The drawing under review shows one solid part. Ordinate dimensions are in mm from its lowest x, y, z. A direction names the side the tool comes from. Round coordinates to 2 decimals unless told otherwise and drop trailing zeros. Loops run counter-clockwise (first coordinate to the right, second up) from the corner with the lowest first, then second, coordinate; pieces in that order, holes last. Notation, with made-up numbers: (69.5, 52.5) -> (98.5, 52.5) arc R24 cw to (98.5, 85.5) -> close; hole circle Ø8 at (0.25, 60.5). An arc over 180 degrees is marked (long way). Use a Markdown table: item, result. Add a question column.
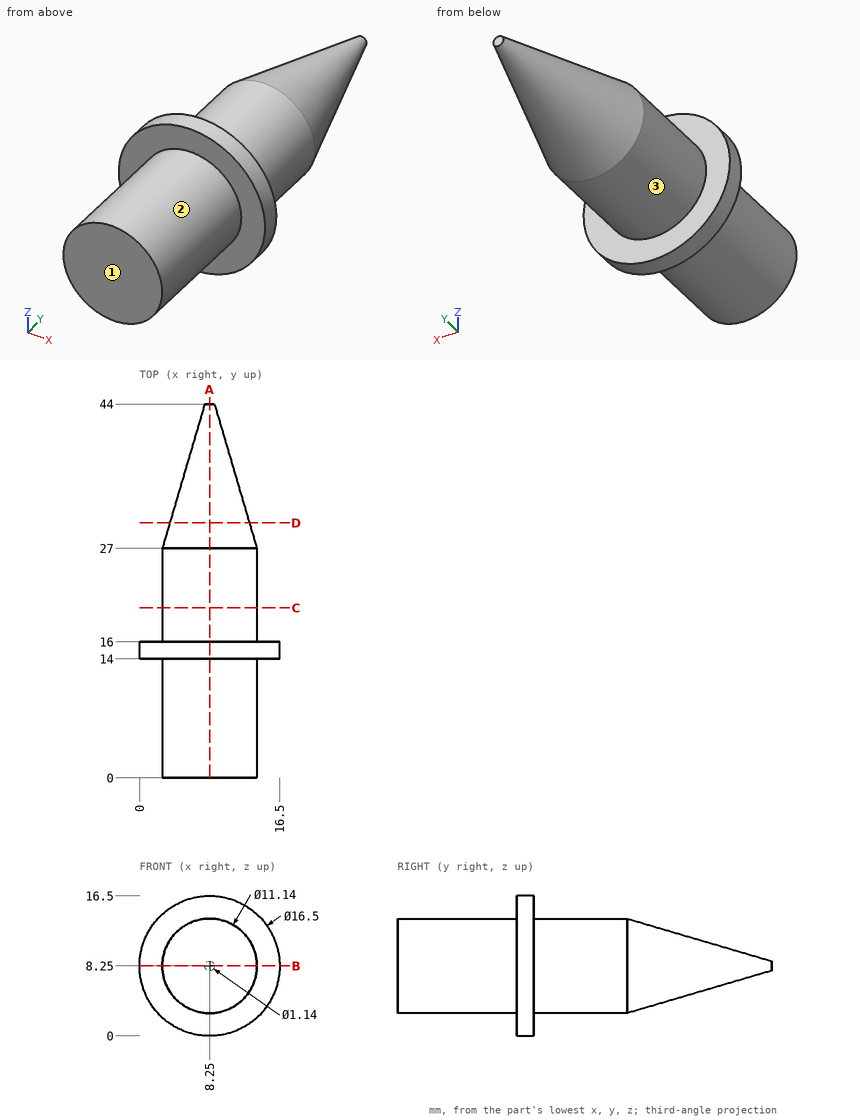
1. Insertion check: P1, Ø2, axis at x = 11, z = 2, coming from the -Y side; P2, Ø6, axis at y = 31.5, z = 2.5, coming from the -X side. Each pin has a flat end and moves straight along its axis. Give the tip position at first contact, or say it passes through.
2. For the marked faces 1, 2 and 3, list the 3-axis set-ups (+Z, -Z, +X, -X, +Y, -Y) from which the entire face can be reached by the end or side of a thin tool; tool diameter is ignored.
3. To check wall thickness, follow probe 1 along Y at (x, z) = (5, 15.25); probe 2 along X at (y, z) = (33, 9.5); probe 3 along X at (y, z) = (12, 5.75). State the ranges of each line that lie inside material, in increasing order. Write a range as from..to.
4. Consider section C-C on y = 20. State the section outline as (x, z) points.
5. Consider section A-A on x = 8.25. State the section outline as (y, z) points.
6. Consider section B-B on z = 8.25. State the section outline as (x, y) points, plus the area to 3 significant figures.
7. Consider section D-D on y = 30. State the section outline as (x, z) points.
Verdict:
| question | item | result |
|---|---|---|
| 1 | P1 | stops at y = 14 |
| 1 | P2 | stops at x = 4.76 |
| 2 | face 1 | +Z, -Z, +X, -X, -Y |
| 2 | face 2 | -Y |
| 2 | face 3 | +Y |
| 3 | probe 1 | y = 14..16 |
| 3 | probe 2 | x = 4.66..11.84 |
| 3 | probe 3 | x = 3.27..13.23 |
| 4 | outline | circle Ø11.14 at (8.25, 8.25) |
| 5 | outline | (0, 2.68) -> (14, 2.68) -> (14, 0) -> (16, 0) -> (16, 2.68) -> (27, 2.68) -> (44, 7.68) -> (44, 8.82) -> (27, 13.82) -> (16, 13.82) -> (16, 16.5) -> (14, 16.5) -> (14, 13.82) -> (0, 13.82) -> close |
| 6 | outline | (0, 14) -> (2.68, 14) -> (2.68, 0) -> (13.82, 0) -> (13.82, 14) -> (16.5, 14) -> (16.5, 16) -> (13.82, 16) -> (13.82, 27) -> (8.82, 44) -> (7.68, 44) -> (2.68, 27) -> (2.68, 16) -> (0, 16) -> close |
| 6 | area | 416 mm² |
| 7 | outline | circle Ø9.38 at (8.25, 8.25) |
